Check sheet for the modelled part. Datum: model origin and axes. Units: mm. A direction names the side the tool comes from. Give positions to 0.01 mm unless a question says otherwise; leave off trailing zeros. Loops run counter-clockwise (first coordinate to the right, second up) from the corner with the lowest first, then second, coordinate; pieces in that order, holes last. Notation, with made-up numbers: (-13.75, 66.5) -> (23.25, 66.5) arc R11 cw to (23.25, 82.5) -> close; hole circle Ø9 at (3, -35.75). An arc over 180 degrees is marked (long way). Write each question's results on one line, items separated by ' | '. Start each with the question number.
Item 1: Cross-section at B-B on y = -20. Enter the section's corners in (x, z).
Item 2: Gauge pin test, flat ends, axial feed: pin 1 Ø1.5 at (x, z) = (25, 9) entering from +Y; pin 2 Ø4 at (x, z) = (-19.5, -4.5) entering from -Y; pin 3 Ø20 at (x, z) = (6, 23.5) entering from +Y; pin 4 Ø2.5 at (y, z) = (28, -12) entering from -X. Record the tip position at first contact, or that the pin passes through.
Item 3: Scan lines: line 1 along X through (y, z) = (3, 19.5); line 2 along X through (y, z) = (31, 27.85); line 3 along Y through (x, z) = (-20, 42). Record each from-to range of solid material in increasing order.
Item 4: Cross-section at D-D on x = 8.5. Enter the section's corners in (y, z), then the cut area to 3 significant figures.
Item 5: Access from +Z, -Z, +X, -X, +Y, -Y to the whole of each face (thin tool, end or side, straight path). Record for faces 1 (the face through (-10, 27, 29)), 2 (the face through (17.5, 29, -12)), 3 (the face through (26.5, -9, 20)), 4 (the face through (30.528, -27.606, 29.92)).
Item 6: Cross-section at C-C on z = 36.5. Enter the section's corners in (x, y).
Item 7: Cross-section at A-A on y = 3.5. Enter the section's corners in (x, z), then the cut area to 3 significant figures.
Item 8: Mould release check, pull along X, two halves, no side actions. Record for faces 5 (the face through (-30, 7, 40)), 6 (the face through (0, 29, 30)), 7 (the face through (-20.35, 31.13, -3.01)): pulls with the +X half, pulls with the -X half, needs draft (parallel to the pull), parting line crosses it, or undercut.
from build123d import *

# Parameters (mm, degrees)
BOSS_EXTRUDE1_DEPTH = 40
SKETCH2_R           = 12.5
CUT_EXTRUDE1_DEPTH  = 4
SKETCH3_R           = 0.75
SKETCH3_R_2         = 4.5
CUT_EXTRUDE2_DEPTH  = 4
SKETCH4_R           = 7.5
CUT_EXTRUDE3_DEPTH  = 14
SKETCH7_W           = 35
SKETCH7_H           = 15
SKETCH7_H_2         = 20
BOSS_EXTRUDE2_DEPTH = 18
SKETCH8_W           = 25
SKETCH8_H           = 55
CUT_EXTRUDE7_DEPTH  = 4
SKETCH9_W           = 20
SKETCH9_H           = 40
CUT_EXTRUDE8_DEPTH  = 3
SKETCH10_R          = 12.5
CUT_EXTRUDE9_DEPTH  = 3
SKETCH11_R          = 4.5
SKETCH11_R_2        = 0.75
CUT_EXTRUDE10_DEPTH = 13
FILLET1_R           = 15
FILLET2_R           = 10
FILLET3_R           = 10


with BuildPart() as part:
    # Sketch1 → Boss-Extrude1 (new body)
    with BuildSketch(Plane.XY):
        Polygon((-26.5, -40), (-26.5, 22), (26.5, 22), (26.5, -40), (32.5, -40), (32.5, 40), (-32.5, 40), (-32.5, -40), align=None)
    extrude(amount=BOSS_EXTRUDE1_DEPTH)

    # Sketch2 → Cut-Extrude1 (cut)
    with BuildSketch(Plane(origin=(32.5, 0, 0), x_dir=(0, 0, -1), z_dir=(1, 0, 0))):
        with Locations((-20, -20)):
            Circle(SKETCH2_R)
    extrude(amount=-CUT_EXTRUDE1_DEPTH, mode=Mode.SUBTRACT)

    # Sketch3 → Cut-Extrude2 (cut)
    with BuildSketch(Plane(origin=(28.5, 0, 0), x_dir=(0, 0, -1), z_dir=(1, 0, 0))):
        with Locations((-20, -12.75)):
            Circle(SKETCH3_R)
        with Locations((-16, -12.75)):
            Circle(SKETCH3_R)
        with Locations((-24, -12.75)):
            Circle(SKETCH3_R)
        with Locations((-20, -20)):
            Circle(SKETCH3_R_2)
        with Locations(Location((-16, -27.25, 0), (0, 0, 90))):
            Circle(SKETCH3_R)
        with Locations(Location((-20, -27.25, 0), (0, 0, 90))):
            Circle(SKETCH3_R)
        with Locations(Location((-24, -27.25, 0), (0, 0, 90))):
            Circle(SKETCH3_R)
    extrude(amount=-CUT_EXTRUDE2_DEPTH, mode=Mode.SUBTRACT)

    # Sketch4 → Cut-Extrude3 (cut)
    with BuildSketch(Plane(origin=(-26.5, 0, 0), x_dir=(0, 0, -1), z_dir=(1, 0, 0))):
        with Locations(Location((-20, -20, 0), (0, 0, 90))):
            Circle(SKETCH4_R)
    extrude(amount=-CUT_EXTRUDE3_DEPTH, mode=Mode.SUBTRACT)

    # Sketch7 → Boss-Extrude2 (add)
    with BuildSketch(Plane(origin=(0, 40, 0), x_dir=(1, 0, 0), z_dir=(0, 1, 0))):
        with Locations((0, 7.5)):
            Rectangle(SKETCH7_W, SKETCH7_H)
        with Locations((0, -50)):
            Rectangle(SKETCH7_W, SKETCH7_H_2)
    extrude(amount=-BOSS_EXTRUDE2_DEPTH)

    # Sketch8 → Cut-Extrude7 (cut)
    with BuildSketch(Plane.XZ.offset(-22)):
        with Locations((0, 29.5)):
            Rectangle(SKETCH8_W, SKETCH8_H)
    extrude(amount=-CUT_EXTRUDE7_DEPTH, mode=Mode.SUBTRACT)

    # Sketch9 → Cut-Extrude8 (cut)
    with BuildSketch(Plane.XZ.offset(-26)):
        with Locations((0, 29.5)):
            Rectangle(SKETCH9_W, SKETCH9_H)
    extrude(amount=-CUT_EXTRUDE8_DEPTH, mode=Mode.SUBTRACT)

    # Sketch10 → Cut-Extrude9 (cut)
    with BuildSketch(Plane(origin=(0, 40, 0), x_dir=(1, 0, 0), z_dir=(0, 1, 0))):
        with Locations(Location((0, -20.6, 0), (0, 0, 270))):
            Circle(SKETCH10_R)
    extrude(amount=-CUT_EXTRUDE9_DEPTH, mode=Mode.SUBTRACT)

    # Sketch11 → Cut-Extrude10 (cut)
    with BuildSketch(Plane(origin=(0, 37, 0), x_dir=(1, 0, 0), z_dir=(0, 1, 0))):
        with Locations(Location((0, -20.6, 0), (0, 0, 270))):
            Circle(SKETCH11_R)
        with Locations(Location((0, -13.35, 0), (0, 0, 270))):
            Circle(SKETCH11_R_2)
        with Locations(Location((4, -13.35, 0), (0, 0, 270))):
            Circle(SKETCH11_R_2)
        with Locations(Location((-4, -13.35, 0), (0, 0, 270))):
            Circle(SKETCH11_R_2)
        with Locations(Location((4, -27.85, 0), (0, 0, 90))):
            Circle(SKETCH11_R_2)
        with Locations(Location((0, -27.85, 0), (0, 0, 90))):
            Circle(SKETCH11_R_2)
        with Locations(Location((-4, -27.85, 0), (0, 0, 90))):
            Circle(SKETCH11_R_2)
    extrude(amount=-CUT_EXTRUDE10_DEPTH, mode=Mode.SUBTRACT)

    # Fillet1
    fillet1_edges = [part.edges().sort_by_distance(p)[0] for p in [
        (-29.5, -40, 0),
        (-29.5, -40, 40),
        (29.5, -40, 40),
        (29.5, -40, 0),
    ]]
    fillet(fillet1_edges, radius=FILLET1_R)

    # Fillet2
    # the kernel refuses this fillet: 10 mm, written as the material it adds along each edge
    with BuildSketch(Plane(origin=(-17.5, 40, 0), x_dir=(-1, 0, 0), z_dir=(0, -1, 0)), Plane(origin=(17.5, 40, 0), x_dir=(0, 0, -1), z_dir=(0, -1, 0))) as fillet2_piece_1:
        with BuildLine():
            CenterArc((FILLET2_R, FILLET2_R), FILLET2_R, 180, 90)
            Line((0, FILLET2_R), (0, 0))
            Line((0, 0), (FILLET2_R, 0))
        make_face()
    extrude(amount=18)
    with BuildSketch(Plane(origin=(-17.5, 40, 40), x_dir=(-1, 0, 0), z_dir=(0, -1, 0)), Plane(origin=(17.5, 40, 40), x_dir=(0, 0, 1), z_dir=(0, -1, 0))) as fillet2_piece_2:
        with BuildLine():
            CenterArc((FILLET2_R, -FILLET2_R), FILLET2_R, 90, 90)
            Line((0, -FILLET2_R), (0, 0))
            Line((0, 0), (FILLET2_R, 0))
        make_face()
    extrude(amount=18)

    # Fillet3
    fillet3_edges = [part.edges().sort_by_distance(p)[0] for p in [
        (0, 40, -15),
        (0, 40, 60),
        (32.5, 40, 20),
        (-32.5, 40, 20),
    ]]
    fillet(fillet3_edges, radius=FILLET3_R)


solid = part.part
Answer sheet:
1) outline: (-32.5, 0) -> (-26.5, 0) -> (-26.5, 12.5) -> (-32.5, 12.5) -> close; (-32.5, 27.5) -> (-26.5, 27.5) -> (-26.5, 40) -> (-32.5, 40) -> close; (26.5, 0) -> (32.5, 0) -> (32.5, 7.5) -> (28.5, 7.5) -> (28.5, 15.5) -> (26.5, 15.5) -> close; (26.5, 24.5) -> (28.5, 24.5) -> (28.5, 32.5) -> (32.5, 32.5) -> (32.5, 40) -> (26.5, 40) -> close
2) pin 1: stops at y = 39.85 | pin 2: stops at y = 22 | pin 3: stops at y = 40 | pin 4: stops at x = -17.5
3) line 1: x = -32.5 to -26.5, 26.5 to 32.5 | line 2: x = -32.45 to -4.75, -3.25 to -0.75, 0.75 to 3.25, 4.75 to 32.45 | line 3: y = 22 to 40
4) outline: (22, -15) -> (30, -15) arc R10 ccw to (40, -5) -> (40, 11.43) -> (37, 11.43) -> (37, 29.77) -> (40, 29.77) -> (40, 50) arc R10 ccw to (30, 60) -> (22, 60) -> (22, 57) -> (26, 57) -> (26, 49.5) -> (29, 49.5) -> (29, 9.5) -> (26, 9.5) -> (26, 2) -> (22, 2) -> close | area: 912 mm²
5) face 1: -Y | face 2: -Z, +X, +Y, -Y | face 3: +Z, -Z, -Y | face 4: +X
6) outline: (-32.5, -34.63) -> (-26.5, -34.63) -> (-26.5, 22) -> (-12.5, 22) -> (-12.5, 26) -> (-10, 26) -> (-10, 29) -> (10, 29) -> (10, 26) -> (12.5, 26) -> (12.5, 22) -> (26.5, 22) -> (26.5, -34.63) -> (32.5, -34.63) -> (32.5, 30) arc R10 ccw to (22.5, 40) -> (-22.5, 40) arc R10 ccw to (-32.5, 30) -> close
7) outline: (-32.5, 0) -> (-26.5, 0) -> (-26.5, 40) -> (-32.5, 40) -> close; (26.5, 0) -> (32.5, 0) -> (32.5, 40) -> (26.5, 40) -> close | area: 480 mm²
8) face 5: needs draft | face 6: undercut | face 7: pulls with the -X half
